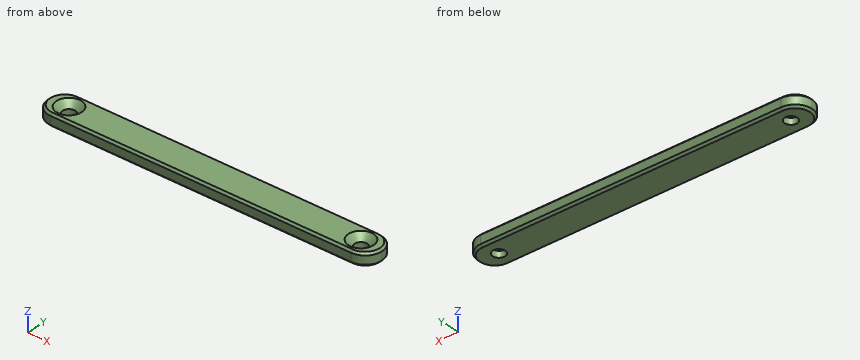
Autodesk Inventor part; units mm, degrees
ref_plane "YZ Plane" through (0, 0, 0) normal (1, 0, 0) x (0, 1, 0)
ref_plane "XZ Plane" through (0, 0, 0) normal (0, 1, 0) x (-1, 0, 0)
ref_plane "XY Plane" through (0, 0, 0) normal (0, 0, 1) x (1, 0, 0)
sketch "Sketch1" plane through (0, 0, 0) normal (0, 0, 1) x (1, 0, 0)
  line L0 (-40, 4) -> (40, 4)
  line L1 (40, 4) -> (40, -4)
  line L2 (40, -4) -> (-40, -4)
  line L3 (-40, -4) -> (-40, 4)
  line L4 (-40, 4) -> (40, -4) construction
  line L5 (40, 4) -> (-40, -4) construction
  line L6 (0, 0) -> (0, 15.184) construction
  circle A0 centre (-35, 0) radius 1.5
  circle A1 centre (35, 0) radius 1.5
  dimension "d0" = 3
  dimension "d1" = 70
  dimension "d2" = 80
  dimension "d3" = 8
extrude "Extrusion1" add sketch "Sketch1" along normal blind 3
chamfer "Chamfer1" distance 1.5 angle 45 2 edges at (-36.5, 0, 3) (33.5, 0, 3)
fillet "Fillet1" radius 4 4 edges at (-40, 4, 1.5) (-40, -4, 1.5) (40, 4, 1.5) (40, -4, 1.5)
chamfer "Chamfer2" distance 0.5 angle 45 8 edges at (0, 4, 0) (-38.8286, 2.8286, 0) (0, -4, 0) (38.8286, 2.8286, 0) (0, 4, 3) (-38.8286, 2.8286, 3) (0, -4, 3) (38.8286, 2.8286, 3)
properties part number "HoldingPlate"
Read the model definition and answer for the solid it produces. Units are mm, in the model's axes. Coordinates: 2 decimals unless noted, no trailing zeros. Loops run counter-clockwise (first coordinate to the right, second up) from the corner with the lowest first, then second, coordinate; pieces in that order, holes last. Notation, with made-up numbers: (-25, 35.25) - (9, 35.25) arc R23 cw to (9, 66.25) - close; hole circle Ø11 at (56, -10). An arc over 180 degrees is marked (long way). Answer in a Markdown table with one row per item.
Q1. Straight lines are drawn through the part: line 1 along Y through (x, z) = (35, 0.95); line 2 along X through (y, z) = (0.25, 2.45); line 3 along Y through (x, z) = (-35, 0.4). For each, find the intervals that lie inside material, in ascending order. Write a range as [from, to].
Here are the results:
| item | result |
|---|---|
| line 1 | y = [-4, -1.5], [1.5, 4] |
| line 2 | x = [-39.99, -37.44], [-32.56, 32.56], [37.44, 39.99] |
| line 3 | y = [-3.9, -1.5], [1.5, 3.9] |
Q2. Find section A-A on x = 35. Write down the section's boundary in (y, z).
Here are the results:
| item | result |
|---|---|
| outline | (-4, 0.5) - (-3.5, 0) - (-1.5, 0) - (-1.5, 1.5) - (-3, 3) - (-3.5, 3) - (-4, 2.5) - close; (1.5, 0) - (3.5, 0) - (4, 0.5) - (4, 2.5) - (3.5, 3) - (3, 3) - (1.5, 1.5) - close |
Q3. Given P1, Ø3.5, axis at x = 35, y = 0, coming from the -Z side, flat-ended and moving along its own axis, determine where the tip first touches the part or whether it passes through.
Here are the results:
| item | result |
|---|---|
| P1 | stops at z = 0 |
Q4. Find section B-B on x = 6.5. Write down the section's boundary in (y, z), plus the area to 3 significant figures.
Here are the results:
| item | result |
|---|---|
| outline | (-4, 0.5) - (-3.5, 0) - (3.5, 0) - (4, 0.5) - (4, 2.5) - (3.5, 3) - (-3.5, 3) - (-4, 2.5) - close |
| area | 23.5 mm^2 |
